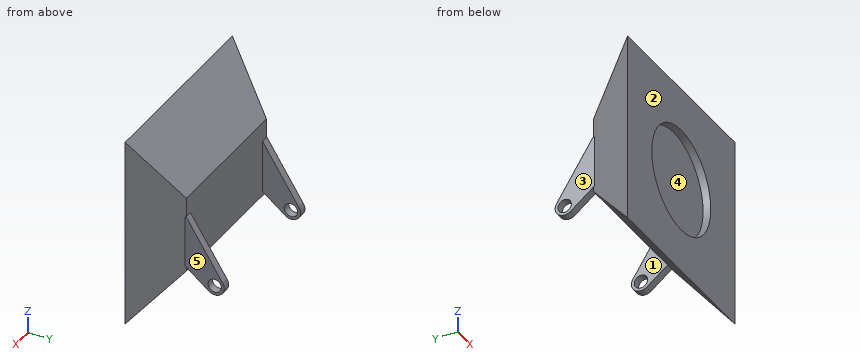
```python
from build123d import *

# Parameters (mm, degrees)
SKETCH4_R           = 137.5
CUT_EXTRUDE1_DEPTH  = 20
BOSS_EXTRUDE1_START = 167.87
BOSS_EXTRUDE1_DEPTH = 20
SKETCH6_R           = 17.5
CUT_EXTRUDE2_DEPTH  = 553.13688256


with BuildPart() as part:
    # Sketch3 → Loft1 section 0
    with BuildSketch(Plane(origin=(0, 125, 0), x_dir=(1, 0, 0), z_dir=(0, 1, 0))):
        with BuildLine():
            Line((186.5, -100), (-186.5, -100))
            Line((-186.5, -100), (-186.5, 100))
            Line((-186.5, 100), (186.5, 100))
            Line((186.5, 100), (186.5, -100))
        make_face()
    # Sketch2 → Loft1 section 1
    with BuildSketch(Plane(origin=(0, 0, 0), x_dir=(1, 0, 0), z_dir=(0, 1, 0))):
        with BuildLine():
            Line((250, -250), (-250, -250))
            Line((-250, -250), (-250, 250))
            Line((-250, 250), (250, 250))
            Line((250, 250), (250, -250))
        make_face()
    loft()

    # Sketch4 → Cut-Extrude1 (cut)
    with BuildSketch(Plane.XZ):
        with Locations(Location((0, 0, 0), (0, 0, 270))):
            Circle(SKETCH4_R)
    extrude(amount=-CUT_EXTRUDE1_DEPTH, mode=Mode.SUBTRACT)

    # Sketch5 → Boss-Extrude1 (add)
    with BuildSketch(Plane(origin=(0, 54.782797639, 0), x_dir=(0, 0, -1), z_dir=(1, 0, 0)).offset(BOSS_EXTRUDE1_START)):
        with BuildLine():
            Line((102.114142863, 166.350579801), (-50, 70.217202361))
            Line((-50, 70.217202361), (11.864642245, -27.672701013))
            Line((11.864642245, -27.672701013), (135.154881767, 129.805922421))
            ThreePointArc((135.154881767, 129.805922421), (134.01437354, 161.983484202), (102.114142863, 166.350579801))
        make_face()
    boss_extrude1 = extrude(amount=BOSS_EXTRUDE1_DEPTH)

    # Sketch6 → Cut-Extrude2 (cut, through all)
    with BuildSketch(Plane(origin=(187.87, 0, 0), x_dir=(0, 0, -1), z_dir=(1, 0, 0))):
        with Locations((115.470053838, 200)):
            Circle(SKETCH6_R)
    cut_extrude2 = extrude(amount=-CUT_EXTRUDE2_DEPTH, mode=Mode.SUBTRACT)

    # Mirror1: Boss-Extrude1, Cut-Extrude2 across plane
    add(boss_extrude1.mirror(Plane(origin=(0, 0, 0), x_dir=(0, 0, 1), z_dir=(1, 0, 0))))
    add(cut_extrude2.mirror(Plane(origin=(0, 0, 0), x_dir=(0, 0, 1), z_dir=(1, 0, 0))), mode=Mode.SUBTRACT)


solid = part.part
```
Check sheet for the modelled part. Datum: model origin and axes. Units: mm. Face numbers are marked on the shaded views. A direction names the side the tool comes from. Coordinates: 2 decimals unless noted, no trailing zeros. Loops run counter-clockwise (first coordinate to the right, second up) from the corner with the lowest first, then second, coordinate; pieces in that order, holes last. Notation, with made-up numbers: M -30,50.25 L -20,50.25 A24 cw -20,77.25 Z; hole C 79.25,2 d4. An arc over 180 degrees is marked long. Answer as a JSON object with one key per item and string values.
1. Access from +Z, -Z, +X, -X, +Y, -Y to the whole of each face (thin tool, end or side, straight path). Record for the marked faces 1 and 2.
Outcome:
{"face 1": "+Z, -Z, +Y", "face 2": "+Z, -Z, +X, -X, -Y"}
2. Sectioned sample at B-B on y = 200. Record the cut outline in (x, z).
Outcome:
{"outline": "M -187.87,-140.47 L -167.87,-140.47 L -167.87,-132.97 L -187.87,-132.97 Z; M -187.87,-97.97 L -167.87,-97.97 L -167.87,-68.67 L -187.87,-68.67 Z; M 167.87,-140.47 L 187.87,-140.47 L 187.87,-132.97 L 167.87,-132.97 Z; M 167.87,-97.97 L 187.87,-97.97 L 187.87,-68.67 L 167.87,-68.67 Z"}
3. Depth check by flat-ended pin: P1, Ø2, axis at x = 132, y = 100, coming from the -Z side; P2, Ø10, axis at x = -75.5, z = -162, coming from the +Y side; P3, Ø5, axis at x = 153.5, y = 90.5, coming from the +Z side. Enter the tip coordinate at first touch or a pass-through.
Outcome:
{"P1": "z = -131.2", "P2": "y = 77.5", "P3": "z = 144.4"}
4. Release check for a two-part mould opening along X. For the marked faces 3, 4 and 5 record: pulls with the +X half, pulls with the -X half, needs draft (parallel to the pull), parting line crosses it, or undercut.
Outcome:
{"face 3": "pulls with the -X half", "face 4": "undercut", "face 5": "pulls with the +X half"}
5. Sectioned sample at A-A on y = 141. Record the cut outline in (x, z).
Outcome:
{"outline": "M -187.87,-101.03 L -167.87,-101.03 L -167.87,24.68 L -187.87,24.68 Z; M 167.87,-101.03 L 187.87,-101.03 L 187.87,24.68 L 167.87,24.68 Z"}
6. Scan lines: L1, parallel to X at y = 201, z = -90.5; L2, parallel to Z at x = 63, y = 68.5; L3, parallel to Y at x = 165.5, z = -58. Record each from-to range of solid material in increasing order. Write a range as from..to.
Outcome:
{"L1": "-187.87..-167.87, 167.87..187.87", "L2": "-167.8..167.8", "L3": "0..125"}
